The model under review builds one solid part; all positions refer to its coordinate system, in mm. A direction names the side the tool comes from. Coordinates: 2 decimals unless noted, no trailing zeros. Loops run counter-clockwise (first coordinate to the right, second up) from the corner with the lowest first, then second, coordinate; pieces in that order, holes last. Notation, with made-up numbers: (46.5, -7.5) - (64.5, -7.5) arc R29 ccw to (64.5, 18.5) - close; hole circle Ø3 at (67.25, 11.25). An arc over 180 degrees is marked (long way). Answer in a Markdown table with one row per item. Add a question column.
(1) We need section A-A on y = 207. Write out the cut boundary in (x, z), plus the area to 3 significant figures.
(2) For P1, Ø10, axis at y = 153, z = -95.5, coming from the -X side; P2, Ø12, axis at x = -537, z = -407.5, coming from the +Y side, all flat-tipped, find the tip position at first contact; note any pin that passes through.
(3) We need section B-B on x = -200.5. Write out the cut boundary in (y, z), plus the area to 3 significant figures.
(4) Mouldability with a two-part tool opening along Z and no side actions: class faces 1 (the flat face through (3, 254, -281)), 2 (the flat face through (-723.9, 125, -426)), 3 (the flat face through (596.9, 125, -99)), 4 (the flat face through (674, 122.5, -242.2)) as +Z half, -Z half, draft (parallel to the pull), parting line (faces both ways), or undercut.
(5) Machinability: for faces 5 (the flat face through (-609.6, 123, -88)), 6 (the flat face through (360, 0, -276)), 7 (the flat face through (609.6, 123, -90)), which of the approach directions +Z, -Z, +X, -X, +Y, -Y give a long, thin tool a straight path to every point of the face, cutting with its end or side? Answer none if there is none.
(6) For line 1 along X through (y, z) = (74.5, -313); line 2 along X through (y, z) = (85.5, -73.5); line 3 along Z through (x, y) = (184, 229.5), list the stretches that pass through material, from the lowest coordinate up.
(7) We need section C-C on z = -97. Write out the cut boundary in (x, y), plus the area to 3 significant figures.
(8) We need section D-D on z = -412. Write out the cut boundary in (x, y), plus the area to 3 significant figures.
from build123d import *

# Parameters (mm, degrees)
BOSS_EXTRUDE1_DEPTH = 254
BOSS_EXTRUDE2_DEPTH = 12.7
SKETCH3_W           = 12.7
SKETCH3_H           = 533.4
BOSS_EXTRUDE3_DEPTH = 254


with BuildPart() as part:
    # Sketch1 → Boss-Extrude1 (new body)
    with BuildSketch(Plane(origin=(0, 0, 0), x_dir=(1, 0, 0), z_dir=(0, 1, 0))):
        Polygon((0, 0), (-609.6, 0), (-609.6, 177.8), (-736.6, 304.8), (-736.6, 558.8), (736.6, 558.8), (736.6, 304.8), (609.6, 177.8), (609.6, 0), align=None)
        Polygon((-723.9, 310.060512242), (-723.9, 546.1), (723.9, 546.1), (723.9, 310.060512242), (596.9, 183.060512242), (596.9, 12.7), (0, 12.7), (-596.9, 12.7), (-596.9, 183.060512242), align=None, mode=Mode.SUBTRACT)
    extrude(amount=BOSS_EXTRUDE1_DEPTH)

    # Sketch2 → Boss-Extrude2 (add)
    with BuildSketch(Plane.XZ):
        Polygon((609.6, -177.8), (609.6, 0), (-609.6, 0), (-609.6, -177.8), (-736.6, -304.8), (-736.6, -558.8), (736.6, -558.8), (736.6, -304.8), align=None)
    extrude(amount=BOSS_EXTRUDE2_DEPTH)

    # Sketch3 → Boss-Extrude3 (add)
    with BuildSketch(Plane(origin=(0, 0, 0), x_dir=(1, 0, 0), z_dir=(0, 1, 0))):
        with Locations((0, 279.4)):
            Rectangle(SKETCH3_W, SKETCH3_H)
    extrude(amount=BOSS_EXTRUDE3_DEPTH)


solid = part.part
Outcome:
| question | item | result |
|---|---|---|
| 1 | outline | (-736.6, -558.8) - (736.6, -558.8) - (736.6, -304.8) - (609.6, -177.8) - (609.6, 0) - (-609.6, 0) - (-609.6, -177.8) - (-736.6, -304.8) - close; hole (-723.9, -546.1) - (-6.35, -546.1) - (-6.35, -12.7) - (-596.9, -12.7) - (-596.9, -183.06) - (-723.9, -310.06) - close; hole (6.35, -546.1) - (723.9, -546.1) - (723.9, -310.06) - (596.9, -183.06) - (596.9, -12.7) - (6.35, -12.7) - close |
| 1 | area | 55,900 mm² |
| 2 | P1 | x = -609.6 |
| 2 | P2 | y = 0 |
| 3 | outline | (-12.7, -558.8) - (254, -558.8) - (254, -546.1) - (0, -546.1) - (0, -12.7) - (254, -12.7) - (254, 0) - (-12.7, 0) - close |
| 3 | area | 13,500 mm² |
| 4 | face 1 | draft |
| 4 | face 2 | undercut |
| 4 | face 3 | undercut |
| 4 | face 4 | +Z half |
| 5 | face 5 | +Z, -X, +Y, -Y |
| 5 | face 6 | +Y |
| 5 | face 7 | +Z, +X, +Y, -Y |
| 6 | line 1 | -736.6 to -723.9, -6.35 to 6.35, 723.9 to 736.6 |
| 6 | line 2 | -609.6 to -596.9, -6.35 to 6.35, 596.9 to 609.6 |
| 6 | line 3 | -558.8 to -546.1, -12.7 to 0 |
| 7 | outline | (-609.6, -12.7) - (609.6, -12.7) - (609.6, 254) - (596.9, 254) - (596.9, 0) - (6.35, 0) - (6.35, 254) - (-6.35, 254) - (-6.35, 0) - (-596.9, 0) - (-596.9, 254) - (-609.6, 254) - close |
| 7 | area | 25,200 mm² |
| 8 | outline | (-736.6, -12.7) - (736.6, -12.7) - (736.6, 254) - (723.9, 254) - (723.9, 0) - (6.35, 0) - (6.35, 254) - (-6.35, 254) - (-6.35, 0) - (-723.9, 0) - (-723.9, 254) - (-736.6, 254) - close |
| 8 | area | 28,400 mm² |
